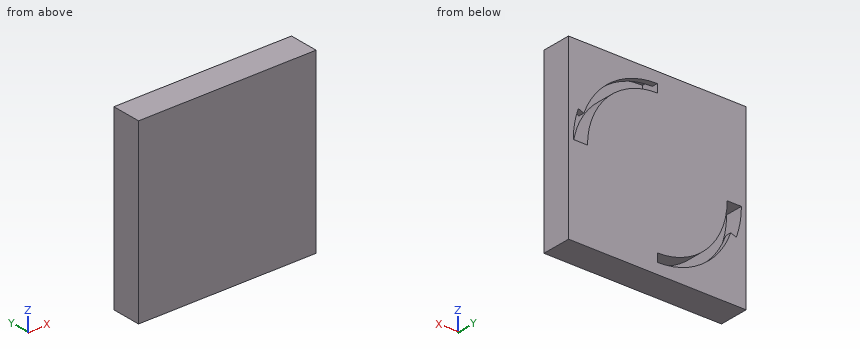
```python
from build123d import *

# Parameters (mm, degrees)
SKETCH1_W           = 30
SKETCH1_H           = 30
BOSS_EXTRUDE1_DEPTH = 5
CUT_REVOLVE2_ANGLE  = 90
SKETCH2_5_W         = 2.4
SKETCH2_5_H         = 3
CUT_REVOLVE3_ANGLE  = 20


with BuildPart() as part:
    # Sketch1 → Boss-Extrude1 (new body)
    with BuildSketch(Plane(origin=(0, 0, 0), x_dir=(1, 0, 0), z_dir=(0, 1, 0))):
        with Locations((15, 15)):
            Rectangle(SKETCH1_W, SKETCH1_H)
    extrude(amount=BOSS_EXTRUDE1_DEPTH)

    # Sketch2 → Cut-Revolve2 (revolve, cut)
    with BuildSketch(Plane.XY.offset(-15)):
        Polygon((1.8, 4), (0.8, 4), (0.8, 2), (3.2, 2), (3.2, 5), (1.8, 5), align=None)
        Polygon((26.8, 2), (29.2, 2), (29.2, 4), (28.2, 4), (28.2, 5), (26.8, 5), align=None)
    revolve(axis=Axis((15, 5, -15), (0, -1, 0)), revolution_arc=CUT_REVOLVE2_ANGLE, mode=Mode.SUBTRACT)

    # Sketch2_5 → Cut-Revolve3 (revolve, cut)
    with BuildSketch(Plane.XY.offset(-15)):
        with Locations((2, 3.5)):
            Rectangle(SKETCH2_5_W, SKETCH2_5_H)
        with Locations((28, 3.5)):
            Rectangle(SKETCH2_5_W, SKETCH2_5_H)
    revolve(axis=Axis((15, 5, -15), (0, -1, 0)), revolution_arc=CUT_REVOLVE3_ANGLE, mode=Mode.SUBTRACT)


solid = part.part
```
Check sheet for the modelled part. Datum: model origin and axes. Units: mm. Round coordinates to 2 decimals unless told otherwise and drop trailing zeros. Loops run counter-clockwise (first coordinate to the right, second up) from the corner with the lowest first, then second, coordinate; pieces in that order, holes last. Notation, with made-up numbers: (0.5, 55.25) -> (49.5, 55.25) arc R5 cw to (49.5, 63.25) -> close; hole circle Ø11 at (-18.75, 23). An arc over 180 degrees is marked (long way). Answer in a Markdown table with one row per item.
Q1. Sectioned sample at B-B on z = -7. Enter the section's corners in (x, y).
Data:
| item | result |
|---|---|
| outline | (0, 0) -> (30, 0) -> (30, 5) -> (25.5, 5) -> (25.5, 4) -> (26.73, 4) -> (26.73, 2) -> (23.67, 2) -> (23.67, 5) -> (0, 5) -> close |
Q2. Sectioned sample at A-A on y = 3.45. Enter the section's corners in (x, z), then the cut area to 3 significant figures.
Data:
| item | result |
|---|---|
| outline | (0, -30) -> (30, -30) -> (30, 0) -> (0, 0) -> close; hole (0.8, -15) arc R14.2 ccw to (15, -29.2) -> (15, -26.8) arc R11.8 cw to (3.2, -15) -> close; hole (15, -3.2) arc R11.8 cw to (26.8, -15) -> (29.2, -15) arc R14.2 ccw to (15, -0.8) -> close |
| area | 802 mm^2 |
Q3. Sectioned sample at C-C on x = 15.5. Enter the section's corners in (y, z), then the cut area to 3 significant figures.
Data:
| item | result |
|---|---|
| outline | (0, -30) -> (5, -30) -> (5, -3.21) -> (2, -3.21) -> (2, -0.81) -> (4, -0.81) -> (4, -1.81) -> (5, -1.81) -> (5, 0) -> (0, 0) -> close |
| area | 144 mm^2 |
Q4. Thickness scan on L1, parallel to Y at x = 27, z = -9.75; L2, parallel to X at y = 3.55, z = -5.25; L3, parallel to X at y = 4.35, z = -4.5. Record the ranges inside material, lowest first.
Data:
| item | result |
|---|---|
| L1 | y = 0 to 2 |
| L2 | x = 0 to 21.65, 25.32 to 30 |
| L3 | x = 0 to 20.38, 23 to 30 |
Q5. Go/stop test with a flat-tipped pin: P1, Ø3, axis at x = 23.5, y = 4.5, coming from the +Z side. Record where the tip stops, or that it passes through.
Data:
| item | result |
|---|---|
| P1 | stops at z = 0 |
Q6. Sectioned sample at D-D on z = -12.75. Enter the section's corners in (x, y), then the cut area to 3 significant figures.
Data:
| item | result |
|---|---|
| outline | (0, 0) -> (30, 0) -> (30, 5) -> (29.02, 5) -> (29.02, 2) -> (26.58, 2) -> (26.58, 5) -> (0, 5) -> close |
| area | 143 mm^2 |
